```python
from build123d import *

# Parameters (mm, degrees)
F1_DEPTH = 152.4
F3_DEPTH = 6.35
F5_DEPTH = 6.35
F7_DEPTH = 101.6
F9_DEPTH = 165.1


with BuildPart() as f1:
    # F0 (on Right) → F1 (new body)
    with BuildSketch(Plane.YZ):
        Polygon((0, 6.35), (0, 0), (203.2, 0), (199.533826, 6.35), align=None)
    extrude(amount=F1_DEPTH)

    # F2 (on face) → F3 (join)
    with BuildSketch(Plane.YZ.offset(152.4)):
        Polygon((0, 0), (203.2, 0), (159.205909, 76.2), (0, 76.2), align=None)
    extrude(amount=F3_DEPTH)

    # F4 (on face) → F5 (join)
    with BuildSketch(Plane(origin=(0, 0, 0), x_dir=(0, -1, 0), z_dir=(-1, 0, 0))):
        Polygon((-159.205909, 76.2), (-203.2, 0), (0, 0), (0, 76.2), align=None)
    extrude(amount=F5_DEPTH)

    # F6 (on face) → F7 (join)
    with BuildSketch(Plane.XZ):
        Polygon((152.4, 76.2), (152.4, 6.35), (0, 6.35), (0, 76.2), (-6.35, 76.2), (-6.35, 0), (158.75, 0), (158.75, 76.2), align=None)
    extrude(amount=F7_DEPTH)

    # F8 (on face) → F9 (cut)
    with BuildSketch(Plane(origin=(-6.35, 0, 0), x_dir=(0, -1, 0), z_dir=(-1, 0, 0))):
        Polygon((57.605909, 76.2), (101.6, 0), (101.6, 76.2), align=None)
    extrude(amount=-F9_DEPTH, mode=Mode.SUBTRACT)


solid = f1.part
```
Geometry: final body of the model. Coordinates: model frame, mm. A direction names the side the tool comes from. Coordinates: 2 decimals unless noted, no trailing zeros. Order: outer loops, then holes, each group sorted by start corner. A loop starts at its lowest first (then second) coordinate and runs counter-clockwise, first axis right, second up. Notation, with made-up numbers: (4.25, -28) -> (59.25, -28) arc R25 ccw to (59.25, -6) -> close; hole circle Ø9 at (-31, -16). An arc over 180 degrees is marked (long way). Answer in a Markdown table with one row per item.
Item 1: Section D-D on z = 22. Output: boundary loops of the cut face in (x, y), plus the area to 3 significant figures.
Return value:
| item | result |
|---|---|
| outline | (-6.35, -88.9) -> (0, -88.9) -> (0, 190.5) -> (-6.35, 190.5) -> close; (152.4, -88.9) -> (158.75, -88.9) -> (158.75, 190.5) -> (152.4, 190.5) -> close |
| area | 3,550 mm² |
Item 2: Section B-B on y = 80.5. Output: boundary loops of the cut face in (x, z).
Return value:
| item | result |
|---|---|
| outline | (-6.35, 0) -> (158.75, 0) -> (158.75, 76.2) -> (152.4, 76.2) -> (152.4, 6.35) -> (0, 6.35) -> (0, 76.2) -> (-6.35, 76.2) -> close |
Item 3: Section C-C on x = 93. Output: boundary loops of the cut face in (y, z), plus the area to 3 significant figures.
Return value:
| item | result |
|---|---|
| outline | (-101.6, 0) -> (203.2, 0) -> (199.53, 6.35) -> (-97.93, 6.35) -> close |
| area | 1,910 mm² |
Item 4: Access query for faces 5 (the flat face through (75.815, -99.053, 4.411)), 6 (the flat face through (152.4, 53, 42)). Directions: +Z, -Z, +X, -X, +Y, -Y. A direction counts if a zero-diameter tool reaches every point of the face in a straight line with its end or side. Return the directions, or none.
Return value:
| item | result |
|---|---|
| face 5 | +Z, +X, -X, -Y |
| face 6 | +Z, +Y, -Y |
Item 5: Draft query along X for faces 1 (the flat face through (158.75, 53, 38)), 2 (the flat face through (156, 52, 76.2)), 3 (the flat face through (77, 53, 6.35)), 4 (the flat face through (-6.35, 53, 39)). Return one class per face: released by +X, released by -X, zero draft, split by the parting line, or undercut.
Return value:
| item | result |
|---|---|
| face 1 | released by +X |
| face 2 | zero draft |
| face 3 | undercut |
| face 4 | released by -X |
Item 6: Section A-A on z = 61.5. Output: boundary loops of the cut face in (x, y), plus the area to 3 significant figures.
Return value:
| item | result |
|---|---|
| outline | (-6.35, -66.09) -> (0, -66.09) -> (0, 167.69) -> (-6.35, 167.69) -> close; (152.4, -66.09) -> (158.75, -66.09) -> (158.75, 167.69) -> (152.4, 167.69) -> close |
| area | 2,970 mm² |
Item 7: Ray query, L1, parallel to X at y = 97, z = 36.5; L2, parallel to Z at x = 37, y = -24; L3, parallel to Y at x = 99.5, z = 3. Return the intervals inside material, ascending.
Return value:
| item | result |
|---|---|
| L1 | x = -6.35 to 0, 152.4 to 158.75 |
| L2 | z = 0 to 6.35 |
| L3 | y = -99.87 to 201.47 |
